Geometry: final body of the model. Coordinates: model frame, mm. A direction names the side the tool comes from. Give positions to 0.01 mm unless a question says otherwise; leave off trailing zeros. Order: outer loops, then holes, each group sorted by start corner. A loop starts at its lowest first (then second) coordinate and runs counter-clockwise, first axis right, second up. Notation, with made-up numbers: (74, -19) - (125, -19) arc R6 cw to (125, -8) - close; hole circle Ø11 at (-30, 61). An arc over 180 degrees is marked (long way). Put each result on its own line as item: value. Start each with the question number.
1. Mould query, pull axis X, two halves, no side actions, for faces 4 (the cylindrical face through (-1.886, 8.493, -0.493)), 5 (the flat face through (0, 0, 4.3)), 6 (the cylindrical face through (-0.596, 2.685, -0.493)). Classes: pulls with the +X half, pulls with the -X half, needs draft (parallel to the pull), parting line crosses it, or undercut.
2. Set-up query: faces 1 (the flat face through (-1, -3, -1)), 2 (the flat face through (0, 0, 0)), 3 (the cylindrical face through (-3, 0, 2)). Return all of +Z, -Z, +X, -X, +Y, -Y with unobstructed straight access to the full face (end or side cutting, diameter ignored); none if empty.
3. Section A-A on z = -0.35. Return the cut outline in (x, y).
4. First-contact query: P1, Ø2, axis at y = -5, z = 3.5, coming from the -X side (3 decimals); P2, Ø5.5, axis at x = -3, y = -4.5, coming from the +Z side; P3, Ø2, axis at x = 2.5, z = 0, coming from the +Y side; P4, Ø3, axis at x = -6, z = 1, coming from the -Y side. Flat tips, straight axial feed; report the tip coordinate or a pass-through.
5. Section B-B on z = 1.7. Return the cut outline in (x, y), plus the area to 3 significant figures.
6. Ray query, line 1 along X through (y, z) = (0, -0.4); line 2 along Z through (x, y) = (-2.25, -7). Return the intervals inside material, ascending. Write a range as from..to.
from build123d import *

# Parameters (mm, degrees)
F0_R     = 9.5
F1_DEPTH = 1
F2_R     = 3
F3_DEPTH = 3.3
F4_R     = 0.8
F5_R     = 5.25
F5_R_2   = 3
F6_DEPTH = 0.3
F7_R     = 8.7
F7_R_2   = 7.75
F7_R_3   = 6.25
F7_R_4   = 5.25
F7_R_5   = 3.75
F7_R_6   = 2.75
F8_DEPTH = 1


# Not quite as in the source:
# - a feature names something its author has since deleted; it is built from what else it names


with BuildPart() as f1:
    # F0 (on Top) → F1 (new body)
    with BuildSketch(Plane.XY):
        Circle(F0_R)
    extrude(amount=F1_DEPTH)

    # F2 (on face) → F3 (join)
    with BuildSketch(Plane.XY.offset(1)):
        Circle(F2_R)
    extrude(amount=F3_DEPTH)

    # F4
    f4_edges = [f1.edges().sort_by_distance(p)[0] for p in [
        (-9.5, 0, 0),
        (-3, 0, 4.3),
    ]]
    fillet(f4_edges, radius=F4_R)

    # F5 (on face) → F6 (join)
    with BuildSketch(Plane.XY.offset(1)):
        Circle(F5_R)
        Circle(F5_R_2, mode=Mode.SUBTRACT)
        Circle(F5_R_2)
    extrude(amount=F6_DEPTH)

    # F7 (on face) → F8 (join)
    with BuildSketch(Plane(origin=(0, 0, 0), x_dir=(1, 0, 0), z_dir=(0, 0, -1))):
        Circle(F7_R)
        Circle(F7_R_2, mode=Mode.SUBTRACT)
        Circle(F7_R_3)
        Circle(F7_R_4, mode=Mode.SUBTRACT)
        Circle(F7_R_5)
        Circle(F7_R_6, mode=Mode.SUBTRACT)
    extrude(amount=F8_DEPTH)


solid = f1.part
Resolved:
1. face 4: parting line crosses it
1. face 5: needs draft
1. face 6: undercut
2. face 1: -Z, +X, -X, +Y, -Y
2. face 2: -Z
2. face 3: +Z
3. outline: circle Ø17.4 at (0, 0); circle Ø12.5 at (0, 0); circle Ø7.5 at (0, 0); hole circle Ø15.5 at (0, 0); hole circle Ø10.5 at (0, 0); hole circle Ø5.5 at (0, 0)
4. P1: through
4. P2: z = 4.16
4. P3: y = 9.33
4. P4: y = -8.37
5. outline: circle Ø6 at (0, 0)
5. area: 28.3 mm^2
6. line 1: -8.7..-7.75, -6.25..-5.25, -3.75..-2.75, 2.75..3.75, 5.25..6.25, 7.75..8.7
6. line 2: 0..1
